Design review of the part built by this model. Coordinates are the model's own, in mm. A direction names the side the tool comes from. Round coordinates to 2 decimals unless told otherwise and drop trailing zeros. Loops run counter-clockwise (first coordinate to the right, second up) from the corner with the lowest first, then second, coordinate; pieces in that order, holes last. Notation, with made-up numbers: M 83,16.5 L 108,16.5 A5 ccw 108,25.5 Z; hole C 19,8 d2. An arc over 180 degrees is marked long. Use a Markdown table: item, result.
from build123d import *

# Parameters (mm, degrees)
BOSS_EXTRUDE1_DEPTH = 8
SKETCH2_R           = 180
BOSS_EXTRUDE2_DEPTH = 1
CUT_EXTRUDE1_REACH  = 10
SKETCH3_R           = 2
CUT_EXTRUDE2_REACH  = 11
SKETCH4_R           = 45


with BuildPart() as part:
    # Sketch1 → Boss-Extrude1 (new body)
    with BuildSketch(Plane.XY):
        Polygon((5, 230), (5, 180), (-5, 180), (-5, 230), (-7, 230), (-157.684812205, 167.584307141), (-159.099025767, 166.170093579), (-123.743686708, 130.814754519), (-130.81475452, 123.743686708), (-166.170093579, 159.099025767), (-167.584307141, 157.684812205), (-230, 7), (-230, 5), (-180, 5), (-180, -5), (-230, -5), (-230, -7), (-167.584307141, -157.684812205), (-166.170093579, -159.099025767), (-130.81475452, -123.743686708), (-123.743686708, -130.81475452), (-159.099025767, -166.170093579), (-157.684812205, -167.584307141), (-7, -230), (-5, -230), (-5, -180), (5, -180), (5, -230), (7, -230), (157.684812205, -167.584307141), (159.099025767, -166.170093579), (123.743686708, -130.814754519), (130.81475452, -123.743686708), (166.170093579, -159.099025767), (167.584307141, -157.684812205), (230, -7), (230, -5), (180, -5), (180, 5), (230, 5), (230, 7), (167.584307141, 157.684812205), (166.170093579, 159.099025767), (130.81475452, 123.743686708), (123.743686708, 130.81475452), (159.099025767, 166.170093579), (157.684812205, 167.584307141), (7, 230), align=None)
    extrude(amount=BOSS_EXTRUDE1_DEPTH)

    # Sketch2 → Boss-Extrude2 (add)
    with BuildSketch(Plane.XY.offset(8)):
        Circle(SKETCH2_R)
    extrude(amount=BOSS_EXTRUDE2_DEPTH)

    # Sketch3 → Cut-Extrude1 (cut, up to next)
    with BuildSketch(Plane.XY.offset(8), mode=Mode.PRIVATE) as cut_extrude1_sk1:
        with Locations((107.397750993, 174.354514299)):
            Circle(SKETCH3_R)
    cut_extrude1_tool1 = extrude(cut_extrude1_sk1.sketch, amount=-CUT_EXTRUDE1_REACH, mode=Mode.PRIVATE) & part.part
    add(cut_extrude1_tool1.solids().sort_by_distance((107.397751, 174.354514, 8))[0], mode=Mode.SUBTRACT)
    # Sketch3 → Cut-Extrude1 (cut, up to next)
    with BuildSketch(Plane.XY.offset(8), mode=Mode.PRIVATE) as cut_extrude1_sk2:
        with Locations((47.34558138, 199.228937402)):
            Circle(SKETCH3_R)
    cut_extrude1_tool2 = extrude(cut_extrude1_sk2.sketch, amount=-CUT_EXTRUDE1_REACH, mode=Mode.PRIVATE) & part.part
    add(cut_extrude1_tool2.solids().sort_by_distance((47.345581, 199.228937, 8))[0], mode=Mode.SUBTRACT)
    # Sketch3 → Cut-Extrude1 (cut, up to next)
    with BuildSketch(Plane.XY.offset(8), mode=Mode.PRIVATE) as cut_extrude1_sk3:
        with Locations((199.228937402, 47.34558138)):
            Circle(SKETCH3_R)
    cut_extrude1_tool3 = extrude(cut_extrude1_sk3.sketch, amount=-CUT_EXTRUDE1_REACH, mode=Mode.PRIVATE) & part.part
    add(cut_extrude1_tool3.solids().sort_by_distance((199.228937, 47.345581, 8))[0], mode=Mode.SUBTRACT)
    # Sketch3 → Cut-Extrude1 (cut, up to next)
    with BuildSketch(Plane.XY.offset(8), mode=Mode.PRIVATE) as cut_extrude1_sk4:
        with Locations((174.354514299, 107.397750993)):
            Circle(SKETCH3_R)
    cut_extrude1_tool4 = extrude(cut_extrude1_sk4.sketch, amount=-CUT_EXTRUDE1_REACH, mode=Mode.PRIVATE) & part.part
    add(cut_extrude1_tool4.solids().sort_by_distance((174.354514, 107.397751, 8))[0], mode=Mode.SUBTRACT)
    # Sketch3 → Cut-Extrude1 (cut, up to next)
    with BuildSketch(Plane.XY.offset(8), mode=Mode.PRIVATE) as cut_extrude1_sk5:
        with Locations((174.354514299, -107.397750993)):
            Circle(SKETCH3_R)
    cut_extrude1_tool5 = extrude(cut_extrude1_sk5.sketch, amount=-CUT_EXTRUDE1_REACH, mode=Mode.PRIVATE) & part.part
    add(cut_extrude1_tool5.solids().sort_by_distance((174.354514, -107.397751, 8))[0], mode=Mode.SUBTRACT)
    # Sketch3 → Cut-Extrude1 (cut, up to next)
    with BuildSketch(Plane.XY.offset(8), mode=Mode.PRIVATE) as cut_extrude1_sk6:
        with Locations((199.228937402, -47.34558138)):
            Circle(SKETCH3_R)
    cut_extrude1_tool6 = extrude(cut_extrude1_sk6.sketch, amount=-CUT_EXTRUDE1_REACH, mode=Mode.PRIVATE) & part.part
    add(cut_extrude1_tool6.solids().sort_by_distance((199.228937, -47.345581, 8))[0], mode=Mode.SUBTRACT)
    # Sketch3 → Cut-Extrude1 (cut, up to next)
    with BuildSketch(Plane.XY.offset(8), mode=Mode.PRIVATE) as cut_extrude1_sk7:
        with Locations((47.34558138, -199.228937402)):
            Circle(SKETCH3_R)
    cut_extrude1_tool7 = extrude(cut_extrude1_sk7.sketch, amount=-CUT_EXTRUDE1_REACH, mode=Mode.PRIVATE) & part.part
    add(cut_extrude1_tool7.solids().sort_by_distance((47.345581, -199.228937, 8))[0], mode=Mode.SUBTRACT)
    # Sketch3 → Cut-Extrude1 (cut, up to next)
    with BuildSketch(Plane.XY.offset(8), mode=Mode.PRIVATE) as cut_extrude1_sk8:
        with Locations((107.397750993, -174.354514299)):
            Circle(SKETCH3_R)
    cut_extrude1_tool8 = extrude(cut_extrude1_sk8.sketch, amount=-CUT_EXTRUDE1_REACH, mode=Mode.PRIVATE) & part.part
    add(cut_extrude1_tool8.solids().sort_by_distance((107.397751, -174.354514, 8))[0], mode=Mode.SUBTRACT)
    # Sketch3 → Cut-Extrude1 (cut, up to next)
    with BuildSketch(Plane.XY.offset(8), mode=Mode.PRIVATE) as cut_extrude1_sk9:
        with Locations((-107.397750993, -174.354514299)):
            Circle(SKETCH3_R)
    cut_extrude1_tool9 = extrude(cut_extrude1_sk9.sketch, amount=-CUT_EXTRUDE1_REACH, mode=Mode.PRIVATE) & part.part
    add(cut_extrude1_tool9.solids().sort_by_distance((-107.397751, -174.354514, 8))[0], mode=Mode.SUBTRACT)
    # Sketch3 → Cut-Extrude1 (cut, up to next)
    with BuildSketch(Plane.XY.offset(8), mode=Mode.PRIVATE) as cut_extrude1_sk10:
        with Locations((-47.34558138, -199.228937402)):
            Circle(SKETCH3_R)
    cut_extrude1_tool10 = extrude(cut_extrude1_sk10.sketch, amount=-CUT_EXTRUDE1_REACH, mode=Mode.PRIVATE) & part.part
    add(cut_extrude1_tool10.solids().sort_by_distance((-47.345581, -199.228937, 8))[0], mode=Mode.SUBTRACT)
    # Sketch3 → Cut-Extrude1 (cut, up to next)
    with BuildSketch(Plane.XY.offset(8), mode=Mode.PRIVATE) as cut_extrude1_sk11:
        with Locations((-199.228937402, -47.34558138)):
            Circle(SKETCH3_R)
    cut_extrude1_tool11 = extrude(cut_extrude1_sk11.sketch, amount=-CUT_EXTRUDE1_REACH, mode=Mode.PRIVATE) & part.part
    add(cut_extrude1_tool11.solids().sort_by_distance((-199.228937, -47.345581, 8))[0], mode=Mode.SUBTRACT)
    # Sketch3 → Cut-Extrude1 (cut, up to next)
    with BuildSketch(Plane.XY.offset(8), mode=Mode.PRIVATE) as cut_extrude1_sk12:
        with Locations((-174.354514299, -107.397750993)):
            Circle(SKETCH3_R)
    cut_extrude1_tool12 = extrude(cut_extrude1_sk12.sketch, amount=-CUT_EXTRUDE1_REACH, mode=Mode.PRIVATE) & part.part
    add(cut_extrude1_tool12.solids().sort_by_distance((-174.354514, -107.397751, 8))[0], mode=Mode.SUBTRACT)
    # Sketch3 → Cut-Extrude1 (cut, up to next)
    with BuildSketch(Plane.XY.offset(8), mode=Mode.PRIVATE) as cut_extrude1_sk13:
        with Locations((-174.354514299, 107.397750993)):
            Circle(SKETCH3_R)
    cut_extrude1_tool13 = extrude(cut_extrude1_sk13.sketch, amount=-CUT_EXTRUDE1_REACH, mode=Mode.PRIVATE) & part.part
    add(cut_extrude1_tool13.solids().sort_by_distance((-174.354514, 107.397751, 8))[0], mode=Mode.SUBTRACT)
    # Sketch3 → Cut-Extrude1 (cut, up to next)
    with BuildSketch(Plane.XY.offset(8), mode=Mode.PRIVATE) as cut_extrude1_sk14:
        with Locations((-199.228937402, 47.34558138)):
            Circle(SKETCH3_R)
    cut_extrude1_tool14 = extrude(cut_extrude1_sk14.sketch, amount=-CUT_EXTRUDE1_REACH, mode=Mode.PRIVATE) & part.part
    add(cut_extrude1_tool14.solids().sort_by_distance((-199.228937, 47.345581, 8))[0], mode=Mode.SUBTRACT)
    # Sketch3 → Cut-Extrude1 (cut, up to next)
    with BuildSketch(Plane.XY.offset(8), mode=Mode.PRIVATE) as cut_extrude1_sk15:
        with Locations((-47.34558138, 199.228937402)):
            Circle(SKETCH3_R)
    cut_extrude1_tool15 = extrude(cut_extrude1_sk15.sketch, amount=-CUT_EXTRUDE1_REACH, mode=Mode.PRIVATE) & part.part
    add(cut_extrude1_tool15.solids().sort_by_distance((-47.345581, 199.228937, 8))[0], mode=Mode.SUBTRACT)
    # Sketch3 → Cut-Extrude1 (cut, up to next)
    with BuildSketch(Plane.XY.offset(8), mode=Mode.PRIVATE) as cut_extrude1_sk16:
        with Locations((-107.397750993, 174.354514299)):
            Circle(SKETCH3_R)
    cut_extrude1_tool16 = extrude(cut_extrude1_sk16.sketch, amount=-CUT_EXTRUDE1_REACH, mode=Mode.PRIVATE) & part.part
    add(cut_extrude1_tool16.solids().sort_by_distance((-107.397751, 174.354514, 8))[0], mode=Mode.SUBTRACT)

    # Sketch4 → Cut-Extrude2 (cut, up to next)
    with BuildSketch(Plane(origin=(0, 0, 0), x_dir=(-1, 0, 0), z_dir=(0, 0, -1)), mode=Mode.PRIVATE) as cut_extrude2_sk1:
        with Locations((-0.557942617, 0.278971308)):
            Circle(SKETCH4_R)
    cut_extrude2_tool1 = extrude(cut_extrude2_sk1.sketch, amount=-CUT_EXTRUDE2_REACH, mode=Mode.PRIVATE) & part.part
    add(cut_extrude2_tool1.solids().sort_by_distance((0.557943, 0.278971, 0))[0], mode=Mode.SUBTRACT)


solid = part.part
1. Machinability: for faces 1 (the face through (-179, 81, 8)), 2 (the face through (-141.17, -148.24, 3.94)), 3 (the face through (-81, -178, 8)), 4 (the face through (83.06, -159.69, 8.49)), which of the approach directions +Z, -Z, +X, -X, +Y, -Y give a long, thin tool a straight path to every point of the face, cutting with its end or side? Answer none if there is none.
Check values:
| item | result |
|---|---|
| face 1 | +Z, -X, +Y |
| face 2 | +Z, -Z |
| face 3 | +Z, -X, -Y |
| face 4 | +Z |
2. Wall thickness on line 1 along X through (y, z) = (-109, 2); line 2 along Y through (x, z) = (-46, 0.75); line 3 along X through (y, z) = (-139, 6.25): over which ranges is each line inside the solid? List them lowest first. Write a range as from..to.
Check values:
| item | result |
|---|---|
| line 1 | x = -187.75..-175.55, -173.16..173.16, 175.55..187.75 |
| line 2 | y = -213.85..-200.71, -197.75..197.75, 200.71..213.85 |
| line 3 | x = -175.32..-146.07, -131.93..131.93, 146.07..175.32 |
3. Insertion check: pin 1 (2.5 mm diameter, centred on x = 0.5, z = 3, fed in from -Y); pin 2 (3 mm diameter, centred on y = -130.5, z = 4.5, fed in from -X); pin 3 (4 mm diameter, centred on x = 213.5, z = 6, fed in from -Y). Each pin has a flat end and moves straight along its axis. Give the tip position at first contact, or say it passes through.
Check values:
| item | result |
|---|---|
| pin 1 | stops at y = -180 |
| pin 2 | stops at x = -179.47 |
| pin 3 | stops at y = -51.66 |
4. Take a section at D-D on z = 2.5. Count the separate pieces of the cut face and the enclosed holes in it, and give its area (3 significant figures).
Check values:
| item | result |
|---|---|
| separate pieces | 1 |
| enclosed holes | 17 |
| area | 143,000 mm² |
5. The part is to be moulded in two halves that separate along X. For faces 5 (the face through (148.74, 141.67, 3.94)), 6 (the face through (81.29, -199.23, 3.94)), 7 (the face through (78, 179, 8)), 8 (the face through (148.24, -141.17, 3.94)), say which applies: pulls with the +X half, pulls with the -X half, needs draft (parallel to the pull), parting line crosses it, or undercut.
Check values:
| item | result |
|---|---|
| face 5 | undercut |
| face 6 | pulls with the +X half |
| face 7 | needs draft |
| face 8 | undercut |
6. Take a section at A-A on x = -189.5. Give the boundary of the cut face in (y, z).
Check values:
| item | result |
|---|---|
| outline | M -104.78,0 L -5,0 L -5,8 L -104.78,8 Z; M 5,0 L 104.78,0 L 104.78,8 L 5,8 Z |
7. Take a section at C-C on x = -92.5. Give the boundary of the cut face in (y, z).
Check values:
| item | result |
|---|---|
| outline | M -194.58,0 L 194.58,0 L 194.58,8 L 154.41,8 L 154.41,9 L -154.41,9 L -154.41,8 L -194.58,8 Z |
8. Take a section at B-B on y = 13. Give the boundary of the cut face in (x, z).
Check values:
| item | result |
|---|---|
| outline | M -227.51,0 L -42.61,0 L -42.61,9 L -179.53,9 L -179.53,8 L -227.51,8 Z; M 43.72,0 L 227.51,0 L 227.51,8 L 179.53,8 L 179.53,9 L 43.72,9 Z |
